Read the model definition and answer for the solid it produces. Units are mm, in the model's axes. A direction names the side the tool comes from. Coordinates: 2 decimals unless noted, no trailing zeros. Write each loop counter-clockwise with the first axis right and the second up, starting at its lowest first coordinate (ties: lowest second). Pieces come first, ordered by that corner, then holes.
Item 1: A tool of negligible diameter and unlimited length cuts with its end or side. For faces 1 (the face through (-5, 12, -42)), 2 (the face through (-5, 12, -55)), 3 (the face through (-5, 12, -35)), 4 (the face through (-2.5, 12, -51)), from which of +Z, -Z, +X, -X, +Y, -Y can it reach the whole face along a straight path? Write none if from no direction.
Item 2: Each of these flat-tipped pins is pushed along its axis until it touches: P1, Ø6.5, axis at y = 16.5, z = -45.5, coming from the +X side; P2, Ø4, axis at x = -30, y = 15, coming from the -Z side; P3, Ø4, axis at x = -4.5, y = 9.5, coming from the -Z side. Where does it stop, or does it pass through?
Item 3: Determine the mould class of faces 5 (the face through (-67.5, 12, -45)), 6 (the face through (-70.806, 1.232, -87.265)), 7 (the face through (-38, 12, -30)) for opening direction Z: released by +Z, released by -Z, zero draft, split by the parting line, or undercut.
Item 4: Straight lines are drawn through the part: probe 1 along Z at (x, y) = (-70, 1.5); probe 2 along X at (y, z) = (1.2, -86); probe 3 along Z at (x, y) = (-53, 15). For each, find the intervals that lie inside material, in ascending order.
Item 5: Section D-D (y = 5.75) is taken. Give the vertices of the cut face in (x, z).
Item 6: Section B-B (x = -5) is taken. Give the vertices of the cut face in (y, z), then the cut area to 3 significant figures.
Item 7: Section C-C (x = -70) is taken. Give the vertices of the cut face in (y, z), then the cut area to 3 significant figures.
Item 8: Section A-A (z = -86) is taken. Give the vertices of the cut face in (x, y).
Autodesk Inventor part; units mm, degrees
ref_plane "YZ Plane" through (0, 0, 0) normal (1, 0, 0) x (0, 1, 0)
ref_plane "XZ Plane" through (0, 0, 0) normal (0, 1, 0) x (-1, 0, 0)
ref_plane "XY Plane" through (0, 0, 0) normal (0, 0, 1) x (1, 0, 0)
sketch "スケッチ1" plane through (0, 0, 0) normal (0, 1, 0) x (-1, 0, 0)
  line L0 (0, 0) -> (75, 0)
  line L1 (75, 0) -> (75, -90)
  line L2 (75, -90) -> (0, -90)
  line L3 (0, -90) -> (0, 0)
  circle A0 centre (70, -4) radius 1.5
  circle A1 centre (70, -86) radius 1.5
  circle A2 centre (5, -4) radius 1.5
  circle A3 centre (5, -86) radius 1.5
  dimension "d0" = 75
  dimension "d1" = 90
  dimension "d4" = 3
  dimension "d5" = 5
  dimension "d6" = 4
  dimension "d7" = 4
  dimension "d8" = 5
  dimension "d9" = 5
  dimension "d10" = 4
  dimension "d11" = 4
extrude "押し出し1" add sketch "スケッチ1" along normal blind 2.5
sketch "スケッチ2" plane through (0, 2.5, 0) normal (0, 1, 0) x (1, 0, 0)
  line L0 (-67.5, 30) -> (-7.5, 30)
  line L1 (-7.5, 30) -> (-7.5, 60)
  line L2 (-7.5, 60) -> (-67.5, 60)
  line L3 (-67.5, 60) -> (-67.5, 30)
  line L4 (-75, 90) -> (-75, 0)
  line L5 (0, 90) -> (-75, 90)
  line L6 (-7.5, 35) -> (-2.5, 35)
  line L7 (-2.5, 35) -> (-2.5, 42)
  line L8 (-2.5, 42) -> (-7.5, 42)
  line L9 (-7.5, 42) -> (-7.5, 35)
  line L10 (-7.5, 48) -> (-2.5, 48)
  line L11 (-2.5, 48) -> (-2.5, 55)
  line L12 (-2.5, 55) -> (-7.5, 55)
  line L13 (-7.5, 55) -> (-7.5, 48)
  point P0 (0, 0)
  point P1 (-67.5, 45)
  point P2 (-75, 45)
  point P3 (-37.5, 60)
  point P4 (-37.5, 90)
  dimension "d13" = 30
  dimension "d14" = 60
  dimension "d15" = 5
  dimension "d16" = 5
  dimension "d17" = 7
  dimension "d18" = 5
extrude "押し出し2" add sketch "スケッチ2" along normal blind 20
equation "\"d7\" = d6"
equation "\"d9\" = d5"
equation "\"d10\" = d6"
equation "\"d11\" = d6"
equation "\"d16\" = d15"
properties part number "control_board"
Established:
1. face 1: +X, +Y
1. face 2: -Z, +X, +Y
1. face 3: +Z, +X, +Y
1. face 4: +Z, -Z, +X, +Y
2. P1: stops at x = -2.5
2. P2: stops at z = -60
2. P3: stops at z = -55
3. face 5: zero draft
3. face 6: undercut
3. face 7: released by +Z
4. probe 1: z = -90 to -87.5, -84.5 to -5.5, -2.5 to 0
4. probe 2: x = -75 to -71.5, -68.5 to -6.5, -3.5 to 0
4. probe 3: z = -60 to -30
5. outline: (-67.5, -60) - (-7.5, -60) - (-7.5, -55) - (-2.5, -55) - (-2.5, -48) - (-7.5, -48) - (-7.5, -42) - (-2.5, -42) - (-2.5, -35) - (-7.5, -35) - (-7.5, -30) - (-67.5, -30) - close
6. outline: (0, -90) - (2.5, -90) - (2.5, -87.5) - (0, -87.5) - close; (0, -84.5) - (2.5, -84.5) - (2.5, -55) - (22.5, -55) - (22.5, -48) - (2.5, -48) - (2.5, -42) - (22.5, -42) - (22.5, -35) - (2.5, -35) - (2.5, -5.5) - (0, -5.5) - close; (0, -2.5) - (2.5, -2.5) - (2.5, 0) - (0, 0) - close
6. area: 490 mm2
7. outline: (0, -90) - (2.5, -90) - (2.5, -87.5) - (0, -87.5) - close; (0, -84.5) - (2.5, -84.5) - (2.5, -5.5) - (0, -5.5) - close; (0, -2.5) - (2.5, -2.5) - (2.5, 0) - (0, 0) - close
7. area: 210 mm2
8. outline: (-75, 0) - (-71.5, 0) - (-71.5, 2.5) - (-75, 2.5) - close; (-68.5, 0) - (-6.5, 0) - (-6.5, 2.5) - (-68.5, 2.5) - close; (-3.5, 0) - (0, 0) - (0, 2.5) - (-3.5, 2.5) - close
